Check sheet for the modelled part. Datum: model origin and axes. Units: mm. A direction names the side the tool comes from. Give positions to 0.01 mm unless a question says otherwise; leave off trailing zeros. Order: outer loops, then holes, each group sorted by start corner. A loop starts at its lowest first (then second) coordinate and runs counter-clockwise, first axis right, second up.
```python
from build123d import *

# Parameters (mm, degrees)
SKETCH_R      = 5
SKETCH_R_2    = 1.25
PAD_DEPTH     = 10
PAD001_DEPTH  = 26
SKETCH003_R   = 2.25
SKETCH003_R_2 = 5
PAD002_DEPTH  = 5


with BuildPart() as part:
    # Sketch → Pad (new body)
    with BuildSketch(Plane.XY):
        with BuildLine():
            Line((0, 11), (23, 11))
            ThreePointArc((33.0374299499, 4.5), (28.9791303716, 9.2330926563), (23, 11))
            Line((23, 4.5), (33.0374299499, 4.5))
            ThreePointArc((23, 4.5), (18.5, 0), (23, -4.5))
            Line((23, -4.5), (33.0374299499, -4.5))
            ThreePointArc((23, -11), (28.9791303716, -9.2330926563), (33.0374299499, -4.5))
            Line((23, -11), (0, -11))
            ThreePointArc((-11, 0), (-7.7781745931, -7.7781745931), (0, -11))
            ThreePointArc((0, 11), (-7.7781745931, 7.7781745931), (-11, 0))
        make_face()
        Circle(SKETCH_R, mode=Mode.SUBTRACT)
        with Locations((-5.6568608175, 5.6568476815)):
            Circle(SKETCH_R_2, mode=Mode.SUBTRACT)
        with Locations((5.6568608175, 5.6568476815)):
            Circle(SKETCH_R_2, mode=Mode.SUBTRACT)
        with Locations((5.6568608175, -5.6568476815)):
            Circle(SKETCH_R_2, mode=Mode.SUBTRACT)
        with Locations((-5.6568345454, -5.6568739536)):
            Circle(SKETCH_R_2, mode=Mode.SUBTRACT)
    extrude(amount=PAD_DEPTH)

    # Sketch002 (on Face16 of Pad) → Pad001 (join)
    with BuildSketch(Plane.XY):
        with BuildLine():
            ThreePointArc((0, 11), (-7.7781745931, 7.7781745931), (-11, 0))
            ThreePointArc((0, 14.5), (-9.1001373616, 9.9811386881), (-11, 0))
            Line((0, 14.5), (7.5, 14.5))
            Line((7.5, 14.5), (11, 11))
            Line((11, 11), (0, 11))
        make_face()
    extrude(amount=PAD001_DEPTH)

    # Sketch003 (on Face11 of Pad001) → Pad002 (join)
    with BuildSketch(Plane.XY.offset(26)):
        with BuildLine():
            Line((0, 11), (11, 11))
            Line((11, 11), (11, 0))
            ThreePointArc((0, 11), (-7.7781745931, -7.7781745931), (11, 0))
        make_face()
        with Locations((-5.6568542391, 5.6568542599)):
            Circle(SKETCH003_R, mode=Mode.SUBTRACT)
        with Locations((5.6568542391, 5.6568542599)):
            Circle(SKETCH003_R, mode=Mode.SUBTRACT)
        with Locations((5.6568542391, -5.6568542599)):
            Circle(SKETCH003_R, mode=Mode.SUBTRACT)
        with Locations((-5.6568542806, -5.6568542184)):
            Circle(SKETCH003_R, mode=Mode.SUBTRACT)
        Circle(SKETCH003_R_2, mode=Mode.SUBTRACT)
    extrude(amount=-PAD002_DEPTH)


solid = part.part
```
(1) Release check for a two-part mould opening along X. For faces 6 (the face through (-7.905, -5.558, 23.535)), 7 (the face through (2, 5, 26)), 8 (the face through (9, 13, 13)) record: released by +X, released by -X, zero draft, split by the parting line, or undercut.
Response values:
face 6: undercut
face 7: zero draft
face 8: released by +X
(2) Material ranges on L1, parallel to Z at x = -9, y = 5; L2, parallel to Z at x = 12.5, y = 5.75; L3, parallel to X at y = 2, z = 5, recorded low to high.
Response values:
L1: z = 0 to 10, 21 to 26
L2: z = 0 to 10
L3: x = -11.37 to -4.58, 4.58 to 18.97
(3) Cross-section at C-C on z = 21.75. Enter the section's corners in (x, y).
Response values:
outline: (-11, 0) arc R11 ccw to (11, 0) - (11, 11) - (7.5, 14.5) - (0, 14.5) arc R11.42 ccw to start; hole circle Ø4.5 at (-5.66, -5.66); hole circle Ø4.5 at (-5.66, 5.66); hole circle Ø10 at (0, 0); hole circle Ø4.5 at (5.66, -5.66); hole circle Ø4.5 at (5.66, 5.66)
(4) Cross-section at B-B on x = 26. Enter the section's corners in (y, z), then the cut area to 3 significant figures.
Response values:
outline: (-10.58, 0) - (-4.5, 0) - (-4.5, 10) - (-10.58, 10) - close; (4.5, 0) - (10.58, 0) - (10.58, 10) - (4.5, 10) - close
area: 122 mm2
(5) Gauge pin test, flat ends, axial feed: pin 1 Ø6 at (x, y) = (23, -8.5) entering from +Z; pin 2 Ø3 at (x, z) = (28, 6) entering from -Y; pin 3 Ø3 at (x, z) = (19, 3.5) entering from +Y. Record the tip position at first contact, or that the pin passes through.
Response values:
pin 1: stops at z = 10
pin 2: stops at y = -10.43
pin 3: stops at y = 11
(6) Cross-section at A-A on y = -0.5. Enter the section's corners in (x, z), then the cut area to 3 significant figures.
Response values:
outline: (-10.99, 0) - (-4.97, 0) - (-4.97, 10) - (-10.99, 10) - close; (-10.99, 21) - (-4.97, 21) - (-4.97, 26) - (-10.99, 26) - close; (4.97, 0) - (18.53, 0) - (18.53, 10) - (4.97, 10) - close; (4.97, 21) - (10.99, 21) - (10.99, 26) - (4.97, 26) - close
area: 256 mm2
(7) Set-up check for faces 1 (the face through (0, -11, 24)), 2 (the face through (11, 6, 24)), 3 (the face through (17, 11, 5)), 4 (the face through (4, 7.18, 23.54)), 5 (the face through (28, 4.5, 5)): record each of +Z, -Z, +X, -X, +Y, -Y from which the full face is reachable in a straight line by a thin tool's end or side.
Response values:
face 1: +Z, -Y
face 2: +Z, +X, +Y, -Y
face 3: +Z, -Z, +X, +Y
face 4: +Z
face 5: +Z, -Z, +X
(8) Cross-section at D-D on z = 13.5. Enter the section's corners in (x, y), then the cut area to 3 significant figures.
Response values:
outline: (-11, 0) arc R11 cw to (0, 11) - (11, 11) - (7.5, 14.5) - (0, 14.5) arc R11.42 ccw to start
area: 74.5 mm2
